Solid Edge part; units mm, degrees
sketch "Sketch1" plane through (0, 0, 0) normal (0, -1, 0) x (1, 0, 0)
  line L0 (0, 20) -> (45.3, 20)
  line L1 (45.3, 20) -> (45.3, -31.15)
  line L2 (45.3, -31.15) -> (25.3, -31.15)
  line L3 (25.3, -31.15) -> (25.3, 0)
  line L4 (25.3, 0) -> (0, 0)
  line L5 (0, 0) -> (0, 20)
  circle A0 centre (10, 10) radius 2.5
extrude "Protrusion1" add sketch "Sketch1" against normal blind 10
sketch "Sketch2" plane through (35.3, 5, -31.15) normal (0, 0, -1) x (1, 0, 0)
  circle A0 centre (0, 0) radius 1
extrude "Cutout1" cut sketch "Sketch2" against normal through all
fillet "Redondeo_1" radius 10 2 edges at (0, 5, 20) (0, 5, 0)
Geometry: final body of the model. Coordinates: model frame, mm. A direction names the side the tool comes from. Coordinates: 2 decimals unless noted, no trailing zeros. Order: outer loops, then holes, each group sorted by start corner. A loop starts at its lowest first (then second) coordinate and runs counter-clockwise, first axis right, second up. Notation, with made-up numbers: (36.5, 83) - (49.5, 83) arc R9 ccw to (49.5, 91) - close; hole circle Ø9 at (-6.75, 53.25). An arc over 180 degrees is marked (long way). Return JSON: item names as keys, results as strings. Group by question number.
1. Cut plane B-B (z = 11.5). Output: boundary loops of the cut face in (x, y), plus the area to 3 significant figures.
2. Material intervals for line 1 along Z through (x, y) = (10, 6.5); line 2 along X through (y, z) = (5, -11); line 3 along X through (y, z) = (4.5, 9), sorted ascending. Write a range as [from, to].
3. Pin query (flat end, axial travel): pin 1 (5 mm diameter, centred on y = 4, z = -15.5, fed in from -X); pin 2 (1 mm diameter, centred on x = 15, y = 4.5, fed in from -Z); pin 3 (4 mm diameter, centred on x = 10, z = 10, fed in from +Y). Return the tip coordinate at first contact, or that it passes through.
4. Pull-direction query (X, two-part tool) for faces 3 (the face through (27, 5, 20)), 4 (the face through (3.01, 5.07, 2.85)), 5 (the face through (34.563, 4.324, -5.933)); classes: pulls with the +X half, pulls with the -X half, needs draft (parallel to the pull), parting line crosses it, or undercut.
5. Set-up query: faces 1 (the face through (2.85, 5.07, 16.99)), 2 (the face through (25.3, 5, -16)). Return all of +Z, -Z, +X, -X, +Y, -Y with unobstructed straight access to the full face (end or side cutting, diameter ignored); none if empty.
6. Cut plane D-D (z = -12). Output: boundary loops of the cut face in (x, y).
7. Cut plane A-A (y = 5). Count the separate pieces of the cut face and the enclosed holes in it, plus the area to 3 significant figures.
Resolved:
{
 "1": {"outline": "(0.11, 0) - (8, 0) - (8, 10) - (0.11, 10) - close; (12, 0) - (45.3, 0) - (45.3, 10) - (12, 10) - close; hole circle Ø2 at (35.3, 5)", "area": "409 mm²"},
 "2": {"line 1": "z = [0, 7.5], [12.5, 20]", "line 2": "x = [25.3, 34.3], [36.3, 45.3]", "line 3": "x = [0.05, 7.71], [12.29, 34.43], [36.17, 45.3]"},
 "3": {"pin 1": "stops at x = 25.3", "pin 2": "stops at z = 0", "pin 3": "passes through"},
 "4": {"face 3": "needs draft", "face 4": "pulls with the -X half", "face 5": "undercut"},
 "5": {"face 1": "+Z, -X, +Y, -Y", "face 2": "-Z, -X, +Y, -Y"},
 "6": {"outline": "(25.3, 0) - (45.3, 0) - (45.3, 10) - (25.3, 10) - close; hole circle Ø2 at (35.3, 5)"},
 "7": {"separate pieces": "2", "enclosed holes": "1", "area": "1,360 mm²"}
}
